from build123d import *

# Parameters (mm, degrees)
BOSS_EXTRUDE1_DEPTH = 50
SKETCH2_W           = 5
SKETCH2_H           = 26.35
BOSS_EXTRUDE2_DEPTH = 20
SKETCH4_W           = 5
SKETCH4_H           = 28.35
BOSS_EXTRUDE3_DEPTH = 20
FILLET2_R           = 2


with BuildPart() as part:
    # Sketch1 → Boss-Extrude1 (new body)
    with BuildSketch(Plane.XY):
        Polygon((-35.507131788, 10.549060403), (-35.507131788, -17.800939597), (-15.507131788, -17.800939597), (-15.507131788, -7.800939597), (-30.507131788, -7.800939597), (-30.507131788, 0.549060403), (-11.107131788, 0.549060403), (-11.107131788, 6.549060403), (2.892868212, 6.549060403), (2.892868212, 0.549060403), (22.292868212, 0.549060403), (22.292868212, -7.800939597), (7.292868212, -7.800939597), (7.292868212, -17.800939597), (27.292868212, -17.800939597), (27.292868212, 10.549060403), align=None)
    extrude(amount=-BOSS_EXTRUDE1_DEPTH)

    # Sketch2 → Boss-Extrude2 (add)
    with BuildSketch(Plane.XY):
        with Locations((-33.007131788, -4.625939597)):
            Rectangle(SKETCH2_W, SKETCH2_H)
        with Locations((24.792868212, -4.625939597)):
            Rectangle(SKETCH2_W, SKETCH2_H)
    extrude(amount=BOSS_EXTRUDE2_DEPTH)

    # Sketch4 → Boss-Extrude3 (add)
    with BuildSketch(Plane(origin=(0, 0, -50), x_dir=(-1, 0, 0), z_dir=(0, 0, -1))):
        with Locations((-24.792868212, -3.625939597)):
            Rectangle(SKETCH4_W, SKETCH4_H)
        with Locations((33.007131788, -3.625939597)):
            Rectangle(SKETCH4_W, SKETCH4_H)
    extrude(amount=BOSS_EXTRUDE3_DEPTH)

    # Fillet2
    fillet2_edges = [part.edges().sort_by_distance(p)[0] for p in [
        (14.792868212, -17.800939597, 0),
        (7.292868212, -12.800939597, 0),
        (-15.507131788, -12.800939597, -50),
        (2.892868212, 3.549060403, 0),
        (-11.107131788, 3.549060403, 0),
        (-15.507131788, -12.800939597, 0),
        (7.292868212, -17.800939597, -25),
        (-15.507131788, -17.800939597, -25),
        (-11.107131788, 3.549060403, -50),
        (2.892868212, 3.549060403, -50),
        (-23.007131788, -17.800939597, 0),
        (-30.507131788, -12.800939597, 0),
        (-30.507131788, -17.800939597, 10),
        (-30.507131788, 4.549060403, 0),
        (7.292868212, -12.800939597, -50),
        (22.292868212, 4.549060403, 0),
        (22.292868212, -12.800939597, 0),
        (22.292868212, -17.800939597, 10),
        (14.792868212, -17.800939597, -50),
        (22.292868212, 5.549060403, -50),
        (22.292868212, -12.800939597, -50),
        (22.292868212, -17.800939597, -60),
        (-23.007131788, -17.800939597, -50),
        (-30.507131788, -12.800939597, -50),
        (-30.507131788, 5.549060403, -50),
        (-30.507131788, -17.800939597, -60),
    ]]
    fillet(fillet2_edges, radius=FILLET2_R)


solid = part.part
Here's how the part is built. I have some questions about the finished solid (model axes, mm). A direction names the side the tool comes from. Coordinates: 2 decimals unless noted, no trailing zeros. Order: outer loops, then holes, each group sorted by start corner. A loop starts at its lowest first (then second) coordinate and runs counter-clockwise, first axis right, second up. Notation, with made-up numbers: (43, 10) - (97, 10) arc R19 cw to (97, 34) - close; hole circle Ø7 at (15.25, 83). An arc over 180 degrees is marked (long way). Use CSV: the item, a comma, the result in double quotes. Start each with the question number.
1. If we mould it in two halves opening along X, with no side actions, what happens to faces 1 (the face through (14.87, -17.23, -49.4)), 2 (the face through (-33, -3, -70))? For each: +X half, -X half, draft (parallel to the pull), parting line (faces both ways), or undercut.
2. For faces 3 (the face through (21.72, 4.61, 0.6)), 4 (the face through (15, -7.801, -25)), 5 (the face through (-15.507, -12, -25)), 6 (the face through (-31.08, -17.2, -61.13)), which set-ups out of +Z, -Z, +X, -X, +Y, -Y let a thin tool reach every point of the face, with its end or its side?
3. Suppose I cut it at B-B on z = 6. List the corners of the cut face in (x, y) for me, then the cut area to 3 significant figures.
4. Please list where these lines run through material, in increasing order: line 1 (X direction, y = -4.75, z = 15.5); line 2 (Y direction, x = 14, z = -11); line 3 (X direction, y = 1, z = -20.5). Write a range as from..to.
5. Suppose I cut it at C-C on x = -20. List the corners of the cut face in (y, z) for me, then the cut area to 3 significant figures.
6. I'm going to push flat-ended pins straight in: pin 1 (9 mm diameter, centred on x = 13, y = -13, fed in from +Z); pin 2 (4 mm diameter, centred on x = -24.5, y = -10, fed in from -Z); pin 3 (20 mm diameter, centred on x = -5, z = -15.5, fed in from -Y); pin 4 (8 mm diameter, centred on x = 2, y = -7, fed in from +Z). Where does each tip first touch, or does it pass through?
7. Suppose I cut it at D-D on z = -47. List the corners of the cut face in (x, y) for me.
8. Suppose I cut it at A-A on y = -2.75. List the corners of the cut face in (x, z) for me.
Output:
1,face 1,"undercut"
1,face 2,"draft"
2,face 3,"+Z, +Y, -Y"
2,face 4,"+Z, -Z"
2,face 5,"+Z, -Z, -Y"
2,face 6,"-Z, -Y"
3,outline,"(-35.51, -17.8) - (-32.51, -17.8) arc R2 ccw to (-30.51, -15.8) - (-30.51, 8.55) - (-35.51, 8.55) - close; (22.29, -15.8) arc R2 ccw to (24.29, -17.8) - (27.29, -17.8) - (27.29, 8.55) - (22.29, 8.55) - close"
3,area,"262 mm2"
4,line 1,"x = -35.51..-30.51, 22.29..27.29"
4,line 2,"y = -17.8..-7.8, 0.55..10.55"
4,line 3,"x = -35.51..-11.11, 2.89..27.29"
5,outline,"(-17.8, -48) arc R2 ccw to (-15.8, -50) - (-7.8, -50) - (-7.8, 0) - (-15.8, 0) arc R2 ccw to (-17.8, -2) - close; (0.55, -50) - (10.55, -50) - (10.55, 0) - (0.55, 0) - close"
5,area,"998 mm2"
6,pin 1,"stops at z = 0"
6,pin 2,"stops at z = -50"
6,pin 3,"stops at y = 0.55"
6,pin 4,"passes through"
7,outline,"(-35.51, -17.8) - (-17.51, -17.8) arc R2 ccw to (-15.51, -15.8) - (-15.51, -7.8) - (-30.51, -7.8) - (-30.51, 0.55) - (-11.11, 0.55) - (-11.11, 6.55) - (2.89, 6.55) - (2.89, 0.55) - (22.29, 0.55) - (22.29, -7.8) - (7.29, -7.8) - (7.29, -15.8) arc R2 ccw to (9.29, -17.8) - (27.29, -17.8) - (27.29, 10.55) - (-35.51, 10.55) - close"
8,outline,"(-35.51, -70) - (-30.51, -70) - (-30.51, 20) - (-35.51, 20) - close; (22.29, -70) - (27.29, -70) - (27.29, 20) - (22.29, 20) - close"
